CAD build for the part. Positions are in the model's coordinates, mm. Face numbers are marked on the shaded views. A direction names the side the tool comes from. Round coordinates to 2 decimals unless told otherwise and drop trailing zeros. Loops run counter-clockwise (first coordinate to the right, second up) from the corner with the lowest first, then second, coordinate; pieces in that order, holes last.
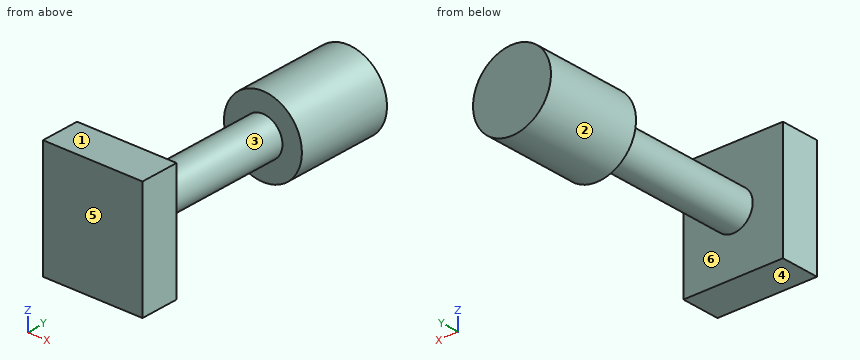
from build123d import *

# Parameters (mm, degrees)
F0_R     = 10
F1_DEPTH = 25
F2_R     = 5
F3_DEPTH = 40
F4_W     = 25.535787
F4_H     = 30
F5_DEPTH = 10


with BuildPart() as f1:
    # F0 (on Front) → F1 (new body)
    with BuildSketch(Plane.XZ):
        with Locations((-28.650001, 26.700001)):
            Circle(F0_R)
    extrude(amount=F1_DEPTH)

    # F2 (on face) → F3 (join)
    with BuildSketch(Plane.XZ.offset(25)):
        with Locations((-28.650001, 26.700001)):
            Circle(F2_R)
    extrude(amount=F3_DEPTH)

    # F4 (on face) → F5 (join)
    with BuildSketch(Plane.XZ.offset(65)):
        with Locations((-28.65, 26.700001)):
            Rectangle(F4_W, F4_H)
    extrude(amount=F5_DEPTH)


solid = f1.part
Item 1: Cut at D-D (z = 15.25). List the corners of the cut face in (x, y).
Verdict:
outline: (-41.42, -75) - (-15.88, -75) - (-15.88, -65) - (-41.42, -65) - close
Item 2: Cut at B-B (z = 34.5). List the corners of the cut face in (x, y), plus the area to 3 significant figures.
Verdict:
outline: (-41.42, -75) - (-15.88, -75) - (-15.88, -65) - (-41.42, -65) - close; (-34.91, -25) - (-22.39, -25) - (-22.39, 0) - (-34.91, 0) - close
area: 568 mm2
Item 3: 3-axis set-ups, long thin cutter, end or side, ignore diameter. For the marked faces 1, 2 and 3: which of +Z, -Z, +X, -X, +Y, -Y reach the whole face in a straight line?
Verdict:
face 1: +Z, +X, -X, +Y, -Y
face 2: +Y
face 3: none
Item 4: Cut at C-C (y = -40). List the corners of the cut face in (x, z).
Verdict:
outline: circle Ø10 at (-28.65, 26.7)
Item 5: Wall check: L1, parallel to Y at x = -31.5, z = 33.75; L2, parallel to Y at x = -17.25, z = 27.75; L3, parallel to X at y = -50.5, z = 26.75. Give the ranges that are in metal, low to high.
Verdict:
L1: y = -75 to -65, -25 to 0
L2: y = -75 to -65
L3: x = -33.65 to -23.65
Item 6: Cut at A-A (x = -36). List the corners of the cut face in (y, z).
Verdict:
outline: (-75, 11.7) - (-65, 11.7) - (-65, 41.7) - (-75, 41.7) - close; (-25, 19.92) - (0, 19.92) - (0, 33.48) - (-25, 33.48) - close
Item 7: Mould opens along Y. For the marked faces 4, 5 and 6 say: released by +Y, released by -Y, zero draft, split by the parting line, or undercut.
Verdict:
face 4: zero draft
face 5: released by -Y
face 6: undercut
Item 8: Flat gauge pins, fed straight in: P1, Ø3, axis at y = -33.5, z = 32.5, coming from the -X side; P2, Ø5, axis at y = -38, z = 21.5, coming from the +X side; P3, Ø4, axis at y = -62.5, z = 28, coming from the +X side; P4, Ø4, axis at x = -36, z = 33.5, coming from the +Y side. Where does each tip first touch, or does it go through?
Verdict:
P1: stops at x = -31.2
P2: stops at x = -24.44
P3: stops at x = -23.65
P4: stops at y = 0
